Input: part model. Units: mm. Frame: model coordinates. A direction names the side the tool comes from. Give positions to 0.01 mm unless a question says otherwise; leave off trailing zeros. Write each loop counter-clockwise with the first axis right and the second up, starting at its lowest first coordinate (ties: lowest second). Pieces come first, ordered by that corner, then holes. Notation, with made-up numbers: (-4.5, 88.25) -> (36.5, 88.25) arc R25 ccw to (36.5, 108.25) -> close; hole circle Ø9 at (-13, 79.25). An arc over 180 degrees is marked (long way). Return JSON: item names as keys, results as strings. Group by question number.
Item 1: Section C-C, the plane y = -5.5. Return loops of the section in (x, z), then the cut area to 3 significant figures.
Item 2: Section B-B, the plane y = -10.5. Count the separate pieces of the cut face and the enclosed holes in it, then the cut area to 3 significant figures.
Item 3: Line query: line 1 (X direction, y = -14, z = 2.5); line 2 (X direction, y = -5.5, z = 5); line 3 (Y direction, x = -1, z = -43.5). Output: solid intervals per line, ascending. Write a range as [from, to].
Item 4: Set-up query: faces 4 (the face through (-17, -3.81, 7)), 5 (the face through (-11, -3.81, -22)), 6 (the face through (-2.719, -22.247, -38.353)), 7 (the face through (-4.438, -12.505, 19.224)), 8 (the face through (5.999, -12.878, -57.456)). Return all of +Z, -Z, +X, -X, +Y, -Y with unobstructed straight access to the full face (end or side cutting, diameter ignored); none if empty.
Item 5: Pin query (flat end, axial travel): P1, Ø8, axis at x = -7, y = -3.5, coming from the -Z side; P2, Ø5, axis at x = -10, y = -14.5, coming from the +Z side; P3, Ø3, axis at x = -4.5, z = 6.5, coming from the +Y side. Return the tip coordinate at first contact, or that it passes through.
Item 6: Section A-A, the plane z = -16.5. Return loops of the section in (x, y).
Item 7: Section D-D, the plane y = -23. Return loops of the section in (x, z) (3 decimals), then the cut area to 3 significant figures.
Item 8: Mould query, pull axis Y, two halves, no side actions, for faces 1 (the face through (-2, -20.656, -45)), 2 (the face through (-17, -21.59, 6)), 3 (the face through (-8, 0, -28)). Classes: released by +Y, released by -Y, zero draft, split by the parting line, or undercut.
from build123d import *

# Parameters (mm, degrees)
F1_DEPTH  = 25.4
F3_DEPTH  = 2.54
F5_DEPTH  = 2.54
F8_DEPTH  = 6.35
F9_DEPTH  = 6.35
F10_D     = 12.7
F10_DEPTH = 50.8
F10_TIP   = 3.8154649308
F13_DEPTH = 50.8
F11_W     = 3.138929677
F11_H     = 9.9252452589
F14_DEPTH = 20.32


with BuildPart() as f1:
    # F0 (on Front) → F1 (new body)
    with BuildSketch(Plane.XZ):
        Polygon((9.3470606522, -38.1387286557), (9.8942405438, -37.2919790531), (-3.1854136077, -28.8397474625), (-3.1854136077, 2.7160348484), (-18.7130940077, 2.7160348484), (-18.7130940077, -49.0474707287), (-3.8916078894, -58.6252953208), (-3.0602029376, -57.3387132966), align=None)
    extrude(amount=F1_DEPTH)

    # F2 (on face) → F3 (join)
    with BuildSketch(Plane.YZ.offset(-3.1854136077)):
        with BuildLine():
            Line((-21.59, 2.7160348484), (-12.7, 2.7160348484))
            Line((-12.7, 2.7160348484), (-12.7, 5.2560348484))
            ThreePointArc((-12.7, 5.2560348484), (-16.2921024484, 6.7439323999), (-17.78, 10.3360348484))
            Line((-17.78, 10.3360348484), (-21.59, 10.3360348484))
            Line((-21.59, 10.3360348484), (-21.59, 2.7160348484))
        make_face()
        with BuildLine():
            Line((-12.7, 5.2560348484), (-12.7, 2.7160348484))
            Line((-12.7, 2.7160348484), (-3.81, 2.7160348484))
            Line((-3.81, 2.7160348484), (-3.81, 10.3360348484))
            Line((-3.81, 10.3360348484), (-7.62, 10.3360348484))
            ThreePointArc((-7.62, 10.3360348484), (-9.1078975516, 6.7439323999), (-12.7, 5.2560348484))
        make_face()
        with BuildLine():
            Line((-21.59, 10.3360348484), (-17.78, 10.3360348484))
            ThreePointArc((-17.78, 10.3360348484), (-12.7, 15.4160348484), (-7.62, 10.3360348484))
            Line((-7.62, 10.3360348484), (-3.81, 10.3360348484))
            ThreePointArc((-3.81, 10.3360348484), (-12.7, 19.2260348484), (-21.59, 10.3360348484))
        make_face()
    extrude(amount=-F3_DEPTH)

    # F4 (on face) → F5 (join)
    with BuildSketch(Plane(origin=(-18.7130940077, 0, 0), x_dir=(0, -1, 0), z_dir=(-1, 0, 0))):
        with BuildLine():
            Line((3.81, 2.7160348484), (12.7, 2.7160348484))
            Line((12.7, 2.7160348484), (12.7, 5.2560348484))
            ThreePointArc((12.7, 5.2560348484), (9.1078975516, 6.7439323999), (7.62, 10.3360348484))
            Line((7.62, 10.3360348484), (3.81, 10.3360348484))
            Line((3.81, 10.3360348484), (3.81, 2.7160348484))
        make_face()
        with BuildLine():
            Line((12.7, 5.2560348484), (12.7, 2.7160348484))
            Line((12.7, 2.7160348484), (21.59, 2.7160348484))
            Line((21.59, 2.7160348484), (21.59, 10.3360348484))
            Line((21.59, 10.3360348484), (17.78, 10.3360348484))
            ThreePointArc((17.78, 10.3360348484), (16.2921024484, 6.7439323999), (12.7, 5.2560348484))
        make_face()
        with BuildLine():
            ThreePointArc((7.62, 10.3360348484), (12.7, 15.4160348484), (17.78, 10.3360348484))
            Line((17.78, 10.3360348484), (21.59, 10.3360348484))
            ThreePointArc((21.59, 10.3360348484), (12.7, 19.2260348484), (3.81, 10.3360348484))
            Line((3.81, 10.3360348484), (7.62, 10.3360348484))
        make_face()
    extrude(amount=-F5_DEPTH)

    # F7 (on face) → F8 (join)
    with BuildSketch(Plane(origin=(-14.0850250818, 0, -21.7962859642), x_dir=(0.8398943412, 0, -0.5427499383), z_dir=(0.5427499383, 0, 0.8398943412))):
        with BuildLine():
            Line((28.5503359742, -17.78), (28.5503359742, -25.4))
            ThreePointArc((28.5503359742, -25.4), (41.2503359742, -12.7), (28.5503359742, 0))
            Line((28.5503359742, 0), (28.5503359742, -7.62))
            ThreePointArc((28.5503359742, -7.62), (32.1424384227, -9.1078975516), (33.6303359742, -12.7))
            ThreePointArc((33.6303359742, -12.7), (32.1424384227, -16.2921024484), (28.5503359742, -17.78))
        make_face()
    extrude(amount=-F8_DEPTH)

    # F6 (on face) → F9 (join)
    with BuildSketch(Plane(origin=(-27.8708735149, 0, -43.129602232), x_dir=(0.8398943412, 0, -0.5427499383), z_dir=(-0.5427499383, 0, -0.8398943412))):
        with BuildLine():
            Line((28.5503359742, 7.62), (28.5503359742, 0))
            ThreePointArc((28.5503359742, 0), (41.2503359742, 12.7), (28.5503359742, 25.4))
            Line((28.5503359742, 25.4), (28.5503359742, 17.78))
            ThreePointArc((28.5503359742, 17.78), (32.1424384227, 16.2921024484), (33.6303359742, 12.7))
            ThreePointArc((33.6303359742, 12.7), (32.1424384227, 9.1078975516), (28.5503359742, 7.62))
        make_face()
    extrude(amount=-F9_DEPTH)

    # F10
    with Locations(Plane(origin=(-27.8708735149, 0, -43.129602232), x_dir=(0.8398943412, 0, -0.5427499383), z_dir=(-0.5427499383, 0, -0.8398943412))):
        with Locations((28.5503359742, 12.7)):
            Hole(F10_D / 2, depth=F10_DEPTH)
            with Locations((0, 0, -(F10_DEPTH + F10_TIP / 2))):  # 118° drill point
                Cone(0, F10_D / 2, F10_TIP, mode=Mode.SUBTRACT)

    # F12 (on face) → F13 (cut)
    with BuildSketch(Plane.XY.offset(2.7160348484)):
        Polygon((-7.7378149144, -17.953234597), (-10.9492538077, -12.7), (-14.1606927009, -17.953234597), (-14.1606927009, -21.59), (-7.7378149144, -21.59), align=None)
        Polygon((-10.9492538077, -12.7), (-14.1606927009, -7.446765403), (-14.1606927009, -17.953234597), align=None)
        Polygon((-7.7378149144, -7.446765403), (-10.9492538077, -12.7), (-7.7378149144, -17.953234597), align=None)
        Polygon((-14.1606927009, -3.81), (-14.1606927009, -7.446765403), (-10.9492538077, -12.7), (-7.7378149144, -7.446765403), (-7.7378149144, -3.81), align=None)
    extrude(amount=-F13_DEPTH, mode=Mode.SUBTRACT)

    # F11 (on face) → F14 (cut)
    with BuildSketch(Plane(origin=(23.9792656255, 0, -15.4956930888), x_dir=(0, 1, 0), z_dir=(0.8398943412, 0, -0.5427499383))):
        with Locations((-22.225, -38.6512237359)):
            Rectangle(F11_W, F11_H)
    extrude(amount=-F14_DEPTH, mode=Mode.SUBTRACT)


solid = f1.part
Answer below:
{
 "1": {"outline": "(-18.71, -49.05) -> (4.9, -64.3) -> (8.34, -58.97) -> (-0.45, -53.29) -> (6.45, -42.63) -> (15.23, -48.3) -> (18.68, -42.97) -> (-3.19, -28.84) -> (-3.19, 15.55) -> (-5.73, 15.55) -> (-5.73, 2.72) -> (-7.74, 2.72) -> (-7.74, -48.08) -> (-14.16, -48.08) -> (-14.16, 2.72) -> (-16.17, 2.72) -> (-16.17, 15.55) -> (-18.71, 15.55) -> close", "area": "941 mm2"},
 "2": {"separate pieces": "5", "enclosed holes": "0", "area": "710 mm2"},
 "3": {"line 1": "x = [-18.71, -14.16], [-7.74, -3.19]", "line 2": "x = [-18.71, -16.17], [-5.73, -3.19]", "line 3": "y = [-25.4, -23.79], [-20.66, -15.33], [-10.07, 0]"},
 "4": {"face 4": "+Z, +X, -X, +Y", "face 5": "+Z", "face 6": "none", "face 7": "+Z, +X, -X", "face 8": "+X, +Y, -Y"},
 "5": {"P1": "stops at z = -59.2", "P2": "stops at z = 2.72", "P3": "stops at y = -3.81"},
 "6": {"outline": "(-18.71, -25.4) -> (-3.19, -25.4) -> (-3.19, 0) -> (-18.71, 0) -> close; hole (-14.16, -21.59) -> (-7.74, -21.59) -> (-7.74, -3.81) -> (-14.16, -3.81) -> close"},
 "7": {"outline": "(-18.713, -49.047) -> (2.349, -62.658) -> (5.795, -57.324) -> (-0.445, -53.292) -> (0.308, -52.127) -> (-16.759, -41.098) -> (-11.372, -32.762) -> (5.695, -43.791) -> (6.448, -42.625) -> (12.688, -46.658) -> (16.134, -41.324) -> (-3.185, -28.84) -> (-3.185, 2.716) -> (-18.713, 2.716) -> close", "area": "961 mm2"},
 "8": {"face 1": "undercut", "face 2": "released by -Y", "face 3": "released by +Y"}
}
